For this review, take the finished solid that the model builds, in its own axes (mm). Face numbers are marked on the shaded views. A direction names the side the tool comes from. Coordinates: 2 decimals unless noted, no trailing zeros. Loops run counter-clockwise (first coordinate to the right, second up) from the corner with the lowest first, then second, coordinate; pieces in that order, holes last. Notation, with made-up numbers: M 58.25,-28 L 92.25,-28 A17 cw 92.25,-3 Z; hole C 31,-25 d4. An arc over 180 degrees is marked long. Put each result on its own line as item: value.
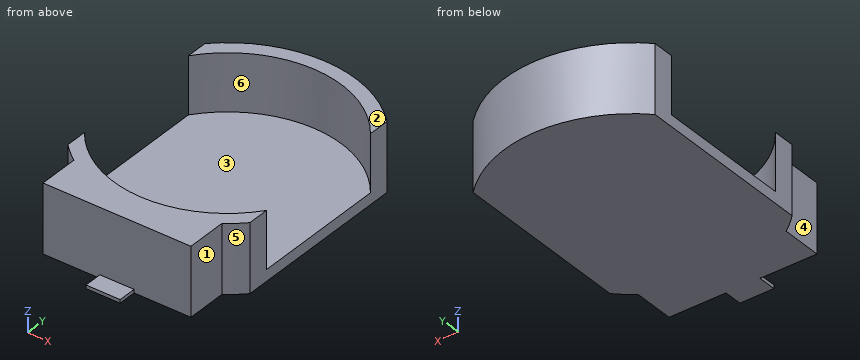
```python
from build123d import *

# Parameters (mm, degrees)
SKETCH1_R           = 11.25
BOSS_EXTRUDE1_DEPTH = 6
SKETCH4_W           = 36
SKETCH4_H           = 45
SKETCH4_W_2         = 16
SKETCH4_H_2         = 25
CUT_EXTRUDE3_DEPTH  = 18.003676073
SKETCH5_W           = 13
SKETCH5_H           = 17
BOSS_EXTRUDE2_DEPTH = 6
SKETCH2_R           = 10
CUT_EXTRUDE4_DEPTH  = 5
SKETCH6_W           = 3
SKETCH6_H           = 0.3
BOSS_EXTRUDE3_DEPTH = 1.6


with BuildPart() as part:
    # Sketch1 → Boss-Extrude1 (new body)
    with BuildSketch(Plane.XY):
        Circle(SKETCH1_R)
    extrude(amount=BOSS_EXTRUDE1_DEPTH)

    # Sketch4 → Cut-Extrude3 (cut, through all)
    with BuildSketch(Plane.XY):
        Rectangle(SKETCH4_W, SKETCH4_H)
        Rectangle(SKETCH4_W_2, SKETCH4_H_2, mode=Mode.SUBTRACT)
    extrude(amount=CUT_EXTRUDE3_DEPTH, mode=Mode.SUBTRACT)

    # Sketch5 → Boss-Extrude2 (add)
    with BuildSketch(Plane.XY):
        with Locations((0, -4.25)):
            Rectangle(SKETCH5_W, SKETCH5_H)
    extrude(amount=BOSS_EXTRUDE2_DEPTH)

    # Sketch2 → Cut-Extrude4 (cut)
    with BuildSketch(Plane.XY.offset(6)):
        Circle(SKETCH2_R)
    extrude(amount=-CUT_EXTRUDE4_DEPTH, mode=Mode.SUBTRACT)

    # Sketch6 → Boss-Extrude3 (add)
    with BuildSketch(Plane.XZ.offset(12.75)):
        with Locations((0, 0.15)):
            Rectangle(SKETCH6_W, SKETCH6_H)
    extrude(amount=BOSS_EXTRUDE3_DEPTH)


solid = part.part
```
(1) For pin 1 (1.8 mm diameter, centred on x = -2.5, z = 2.5, fed in from -Y); pin 2 (3 mm diameter, centred on y = -11, z = 2.5, fed in from -X); pin 3 (3 mm diameter, centred on x = 3.5, z = 3.5, fed in from +Y), all flat-tipped, find the tip position at first contact; note any pin that passes through.
Determined:
pin 1: stops at y = -12.75
pin 2: stops at x = -6.5
pin 3: stops at y = 11.07
(2) Add section B-B (y = -7). Write out the cut boundary in (x, z), plus the area to 3 significant figures.
Determined:
outline: M -8,0 L 8,0 L 8,6 L 7.14,6 L 7.14,1 L -7.14,1 L -7.14,6 L -8,6 Z
area: 24.6 mm^2
(3) Add section D-D (y = 2.75). Write out the cut boundary in (x, z).
Determined:
outline: M -8,0 L 8,0 L 8,1 L -8,1 Z
(4) Add section C-C (x = 6.25). Write out the cut boundary in (y, z).
Determined:
outline: M -12.75,0 L 9.35,0 L 9.35,6 L 7.81,6 L 7.81,1 L -7.81,1 L -7.81,6 L -12.75,6 Z
(5) Draft analysis for pull direction Y (two halves, no side actions). For the marked faces 4, 5 and 6, state which applies: +Y half, -Y half, draft (parallel to the pull), parting line (faces both ways), or undercut.
Determined:
face 4: draft
face 5: -Y half
face 6: undercut
(6) Tool access review of the marked faces 1, 2 and 3: name each direction out of +Z, -Z, +X, -X, +Y, -Y from which nothing blocks a thin tool from reaching the whole face with its end or side.
Determined:
face 1: +Z, -Z, +X, -Y
face 2: +Z, +X, -X, +Y, -Y
face 3: +Z
(7) Add section A-A (z = 1.9). Write out the cut boundary in (x, y).
Determined:
outline: M -8,-7.91 A11.25 ccw -6.5,-9.18 L -6.5,-12.75 L 6.5,-12.75 L 6.5,-9.18 A11.25 ccw 8,-7.91 L 8,-6 A10 cw -8,-6 Z; M -8,6 A10 cw 8,6 L 8,7.91 A11.25 ccw -8,7.91 Z
(8) Wall thickness on line 1 along Y through (x, z) = (2, 3.8); line 2 along X through (y, z) = (7.25, 4.3); line 3 along Z through (x, y) = (-1, 8.5): over which ranges is each line inside the solid? List them lowest first. Write a range as [from, to].
Determined:
line 1: y = [-12.75, -9.8], [9.8, 11.07]
line 2: x = [-8, -6.89], [6.89, 8]
line 3: z = [0, 1]
